from build123d import *

# Parameters (mm, degrees)
SKETCH1_W                 = 88.9
SKETCH1_H                 = 88.9
SKETCH1_R                 = 3.937
BOSS_EXTRUDE1_DEPTH       = 9.906
SKETCH2_W                 = 56.134
SKETCH2_H                 = 48.26
BOSS_EXTRUDE2_DEPTH       = 19.05
SKETCH3_W                 = 66.294
SKETCH3_H                 = 58.42
BOSS_EXTRUDE3_DEPTH       = 63.246
SKETCH4_W                 = 47.752
SKETCH4_H                 = 25.4
CUT_EXTRUDE1_DEPTH        = 76.2
SKETCH5_W                 = 60.452
SKETCH5_H                 = 38.1
CUT_EXTRUDE2_DEPTH        = 3.302
SKETCH6_R                 = 6.35
CUT_EXTRUDE3_DEPTH        = 129.445730614
SKETCH6_3_R               = 8.763
SKETCH6_3_R_2             = 6.35
CUT_EXTRUDE4_DEPTH        = 6.35
SKETCH8_R                 = 6.35
CUT_EXTRUDE5_DEPTH        = 127.106331736
FILLET1_R                 = 3.302
FILLET2_R                 = 3.302
FILLET3_R                 = 7.112
F_4_40_TAPPED_HOLE2_D     = 2.2606
F_4_40_TAPPED_HOLE2_DEPTH = 8.89
F_4_40_TAPPED_HOLE2_TIP   = 0.679152758


with BuildPart() as part:
    # Sketch1 → Boss-Extrude1 (new body)
    with BuildSketch(Plane(origin=(0, 0, 0), x_dir=(1, 0, 0), z_dir=(0, 1, 0))):
        Rectangle(SKETCH1_W, SKETCH1_H)
        with Locations(Location((-34.925, 34.925, 0), (0, 0, 270))):
            Circle(SKETCH1_R, mode=Mode.SUBTRACT)
        with Locations(Location((-34.925, -34.925, 0), (0, 0, 270))):
            Circle(SKETCH1_R, mode=Mode.SUBTRACT)
        with Locations(Location((34.925, 34.925, 0), (0, 0, 270))):
            Circle(SKETCH1_R, mode=Mode.SUBTRACT)
        with Locations(Location((34.925, -34.925, 0), (0, 0, 270))):
            Circle(SKETCH1_R, mode=Mode.SUBTRACT)
    extrude(amount=BOSS_EXTRUDE1_DEPTH)

    # Sketch2 → Boss-Extrude2 (add)
    with BuildSketch(Plane(origin=(0, 9.906, 0), x_dir=(1, 0, 0), z_dir=(0, 1, 0))):
        Rectangle(SKETCH2_W, SKETCH2_H)
    extrude(amount=BOSS_EXTRUDE2_DEPTH)

    # Sketch3 → Boss-Extrude3 (add)
    with BuildSketch(Plane(origin=(0, 28.956, 0), x_dir=(1, 0, 0), z_dir=(0, 1, 0))):
        Rectangle(SKETCH3_W, SKETCH3_H)
    extrude(amount=BOSS_EXTRUDE3_DEPTH)

    # Sketch4 → Cut-Extrude1 (cut)
    with BuildSketch(Plane.XZ):
        Rectangle(SKETCH4_W, SKETCH4_H)
    extrude(amount=-CUT_EXTRUDE1_DEPTH, mode=Mode.SUBTRACT)

    # Sketch5 → Cut-Extrude2 (cut)
    with BuildSketch(Plane.XZ):
        Rectangle(SKETCH5_W, SKETCH5_H)
    extrude(amount=-CUT_EXTRUDE2_DEPTH, mode=Mode.SUBTRACT)

    # Sketch6 → Cut-Extrude3 (cut, through all)
    with BuildSketch(Plane.ZY.offset(33.147)):
        with Locations((0, 67.31)):
            Circle(SKETCH6_R)
    extrude(amount=-CUT_EXTRUDE3_DEPTH, mode=Mode.SUBTRACT)

    # Sketch6_3 → Cut-Extrude4 (cut)
    with BuildSketch(Plane.ZY.offset(33.147)):
        with Locations((0, 67.31)):
            Circle(SKETCH6_3_R)
        with Locations((0, 67.31)):
            Circle(SKETCH6_3_R_2, mode=Mode.SUBTRACT)
    cut_extrude4 = extrude(amount=-CUT_EXTRUDE4_DEPTH, mode=Mode.SUBTRACT)

    # Mirror1: Cut-Extrude4 across plane
    add(cut_extrude4.mirror(Plane(origin=(0, 0, 0), x_dir=(0, 0, 1), z_dir=(1, 0, 0))), mode=Mode.SUBTRACT)

    # Sketch8 → Cut-Extrude5 (cut, through all)
    with BuildSketch(Plane(origin=(0, 0, -29.21), x_dir=(-1, 0, 0), z_dir=(0, 0, -1))):
        with Locations((0, 37.084)):
            Circle(SKETCH8_R)
    extrude(amount=-CUT_EXTRUDE5_DEPTH, mode=Mode.SUBTRACT)

    # Fillet1
    fillet1_edges = [part.edges().sort_by_distance(p)[0] for p in [
        (-44.45, 9.906, 0),
        (0, 9.906, 44.45),
        (44.45, 9.906, 0),
        (33.147, 60.579, 29.21),
        (33.147, 60.579, -29.21),
        (-33.147, 60.579, -29.21),
        (-33.147, 60.579, 29.21),
        (33.147, 92.202, 0),
        (0, 92.202, -29.21),
        (-33.147, 92.202, 0),
        (0, 92.202, 29.21),
        (0, 9.906, -44.45),
    ]]
    fillet(fillet1_edges, radius=FILLET1_R)

    # Fillet2
    fillet2_edges = [part.edges().sort_by_distance(p)[0] for p in [
        (30.226, 1.651, 19.05),
        (30.226, 1.651, -19.05),
        (-30.226, 1.651, -19.05),
        (-30.226, 1.651, 19.05),
    ]]
    fillet(fillet2_edges, radius=FILLET2_R)

    # Fillet3
    fillet3_edges = [part.edges().sort_by_distance(p)[0] for p in [
        (23.876, 39.751, 12.7),
        (23.876, 39.751, -12.7),
        (-23.876, 39.751, -12.7),
        (-23.876, 39.751, 12.7),
    ]]
    fillet(fillet3_edges, radius=FILLET3_R)

    # 4-40 Tapped Hole2
    with Locations(Plane(origin=(0, 3.302, 0), x_dir=(-1, 0, 0), z_dir=(0, -1, 0))):
        with Locations((26.289, -15.08840493), (-26.289, -15.08840493), (-26.289, 15.08840493), (26.289, 15.08840493)):
            Hole(F_4_40_TAPPED_HOLE2_D / 2, depth=F_4_40_TAPPED_HOLE2_DEPTH)
            with Locations((0, 0, -(F_4_40_TAPPED_HOLE2_DEPTH + F_4_40_TAPPED_HOLE2_TIP / 2))):  # 118° drill point
                Cone(0, F_4_40_TAPPED_HOLE2_D / 2, F_4_40_TAPPED_HOLE2_TIP, mode=Mode.SUBTRACT)


solid = part.part
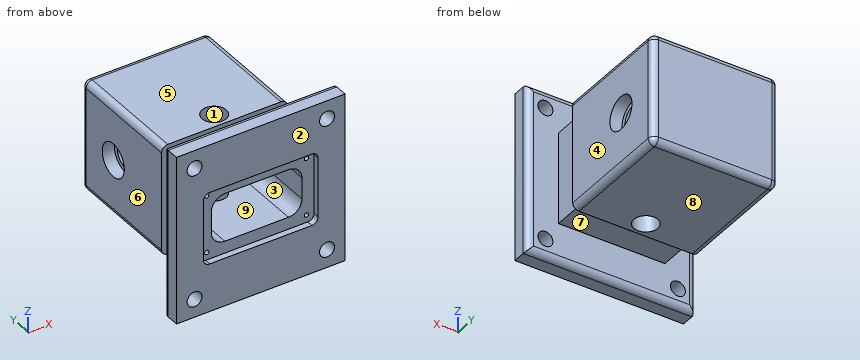
Geometry: final body of the model. Coordinates: model frame, mm. Face numbers are marked on the shaded views. A direction names the side the tool comes from. Give positions to 0.01 mm unless a question says otherwise; leave off trailing zeros. Order: outer loops, then holes, each group sorted by start corner. A loop starts at its lowest first (then second) coordinate and runs counter-clockwise, first axis right, second up. Notation, with made-up numbers: (72.5, -4.5) -> (106.5, -4.5) arc R24 cw to (106.5, 28.5) -> close; hole circle Ø8 at (75.5, 20). An arc over 180 degrees is marked (long way). Write each question's results on one line, items separated by ' | '.
1) Cut plane A-A (x = 0). Give the number of separate pieces and of enclosed holes in the cut face, and give its area (3 significant figures).
Geometry says:
separate pieces: 3 | enclosed holes: 0 | area: 3,090 mm²
2) First-contact query: pin 1 Ø1 at (x, y) = (-2, 24.5) entering from +Z; pin 2 Ø12.5 at (y, z) = (23, 2) entering from +X; pin 3 Ø10 at (x, y) = (-7, 33.5) entering from -Z; pin 4 Ø1 at (x, z) = (-30, -19) entering from +Y. Flat tips, straight axial feed; report the tip coordinate or a pass-through.
Geometry says:
pin 1: stops at z = 24.13 | pin 2: stops at x = 33.15 | pin 3: stops at z = -29.21 | pin 4: stops at y = 92.2
3) Line query: line 1 along Z through (x, y) = (-5, 67); line 2 along Y through (x, z) = (0, -21); line 3 along X through (y, z) = (16, -5). Output: solid intervals per line, ascending.
Geometry says:
line 1: z = -29.21 to -12.7, 12.7 to 29.21 | line 2: y = 0 to 30.73, 43.43 to 92.2 | line 3: x = -28.07 to -23.88, 23.88 to 28.07
4) Set-up query: the marked faces 5, 6, 7, 8 and 9. Return all of +Z, -Z, +X, -X, +Y, -Y with unobstructed straight access to the full face (end or side cutting, diameter ignored); none if empty.
Geometry says:
face 5: +Z, +X, -X, +Y | face 6: +Z, -Z, -X, +Y | face 7: -Z, +X, -X | face 8: -Z, +X, -X, +Y | face 9: -Y
5) Draft query along X for the marked faces 1, 2, 3 and 4. Return one class per face: released by +X, released by -X, zero draft, split by the parting line, or undercut.
Geometry says:
face 1: undercut | face 2: zero draft | face 3: undercut | face 4: released by +X
6) Cut plane B-B (y = 23). Output: boundary loops of the cut face in (x, z).
Geometry says:
outline: (-28.07, -24.13) -> (28.07, -24.13) -> (28.07, 24.13) -> (-28.07, 24.13) -> close; hole (-23.88, -5.59) arc R7.11 ccw to (-16.76, -12.7) -> (16.76, -12.7) arc R7.11 ccw to (23.88, -5.59) -> (23.88, 5.59) arc R7.11 ccw to (16.76, 12.7) -> (-16.76, 12.7) arc R7.11 ccw to (-23.88, 5.59) -> close
7) Cut plane D-D (y = 80). Output: boundary loops of the cut face in (x, z) (3 decimals), and give its area (3 significant figures).
Geometry says:
outline: (-33.147, -25.908) arc R3.302 ccw to (-29.845, -29.21) -> (29.845, -29.21) arc R3.302 ccw to (33.147, -25.908) -> (33.147, 25.908) arc R3.302 ccw to (29.845, 29.21) -> (-29.845, 29.21) arc R3.302 ccw to (-33.147, 25.908) -> close | area: 3,860 mm²
